Autodesk Inventor part; units mm, degrees
ref_plane "YZ Plane" through (0, 0, 0) normal (1, 0, 0) x (0, 1, 0)
ref_plane "XZ Plane" through (0, 0, 0) normal (0, 1, 0) x (-1, 0, 0)
ref_plane "XY Plane" through (0, 0, 0) normal (0, 0, 1) x (1, 0, 0)
sketch "Sketch1" plane through (0, 0, 0) normal (0, 0, 1) x (1, 0, 0)
  line L0 (0, 0) -> (58, 0)
  line L1 (58, 0) -> (58, 178)
  line L2 (58, 178) -> (0, 178)
  line L3 (0, 178) -> (0, 0)
  dimension "d0" = 58
  dimension "d1" = 178
extrude "Extrusion1" add sketch "Sketch1" along normal blind 60
shell "Shell1" thickness 3 removed faces 1 at (19.3333, 118.6667, 0)
sketch "Sketch2" plane through (0, 0, 60) normal (0, 0, 1) x (1, 0, 0)
  line L0 (3, 3) -> (55, 3)
  line L1 (3, 3) -> (8, 3)
  line L2 (8, 3) -> (8, 6.3)
  line L3 (55, 3) -> (55, 175)
  line L4 (55, 175) -> (55, 170)
  line L5 (55, 170) -> (51.7, 170)
  line L6 (48.3, 170) -> (9.7, 170)
  line L7 (8, 168.3) -> (8, 9.7)
  line L8 (9.7, 8) -> (48.3, 8)
  line L9 (50, 9.7) -> (50, 168.3)
  circle A0 centre (8, 8) radius 1.7
  line L10 (9.7, 8) -> (13, 8)
  line L11 (8, 9.7) -> (8, 13)
  line L12 (8, 13) -> (13, 13)
  line L13 (13, 13) -> (13, 8)
  line L14 (29, 8) -> (29, 9.7)
  circle A1 centre (50, 8) radius 1.7
  line L15 (48.3, 8) -> (45, 8)
  line L16 (50, 9.7) -> (50, 13)
  line L17 (50, 13) -> (45, 13)
  line L18 (45, 13) -> (45, 8)
  line L19 (50, 89) -> (45, 89)
  circle A2 centre (8, 170) radius 1.7
  line L20 (9.7, 170) -> (13, 170)
  line L21 (8, 168.3) -> (8, 165)
  line L22 (8, 165) -> (13, 165)
  line L23 (13, 165) -> (13, 170)
  circle A3 centre (50, 170) radius 1.7
  line L24 (48.3, 170) -> (45, 170)
  line L25 (50, 168.3) -> (50, 165)
  line L26 (45, 165) -> (45, 170)
  line L27 (50, 165) -> (45, 165)
  point P0 (0, 0)
  point P1 (58, 0)
  point P2 (58, 178)
  point P3 (0, 178)
  point P4 (50, 6.3)
  point P5 (8, 171.7)
  point P6 (50, 171.7)
  dimension "d29" = 5
  dimension "d31" = 5
  dimension "d32" = 5
  dimension "d33" = 3.4
  dimension "d34" = 3.3
  dimension "d35" = 3.3
extrude "Extrusion4" cut sketch "Sketch2" against normal blind 3 contours A0 | A3 | L7 L22 L23 L6 L26 L27 L9 L17 L18 L8 L13 L12 | A2 | A1
sketch "Sketch4" plane through (58, 0, 0) normal (1, 0, 0) x (0, 0, -1)
  line L0 (0, 3) -> (-57, 3)
  line L1 (0, 3) -> (-3, 3)
  line L2 (-3, 3) -> (-23, 3)
  line L3 (-23, 3) -> (-23, 103)
  line L4 (-23, 103) -> (-3, 103)
  line L5 (-3, 103) -> (-3, 3)
  line L6 (-23, 3) -> (-23, 13)
  line L7 (-23, 13) -> (-3, 13)
  point P0 (0, 0)
  dimension "d38" = 3
  dimension "d39" = 20
  dimension "d40" = 100
  dimension "d41" = 10
extrude "Extrusion5" cut sketch "Sketch4" against normal blind 4 contours L7 L3 L4 L5
sketch "Sketch5" plane through (0, 178, 0) normal (0, 1, 0) x (1, 0, 0)
  line L0 (55, 0) -> (3, 0)
  line L1 (29, 0) -> (29, -60)
  line L2 (58, -60) -> (0, -60)
  line L3 (55, 0) -> (55, -57)
  circle A0 centre (43.5, -30) radius 2.5
  circle A1 centre (14.5, -30) radius 2.5
  point P0 (0, 0)
  dimension "d44" = 5
extrude "Extrusion6" cut sketch "Sketch5" against normal blind 4
properties part number "port side"
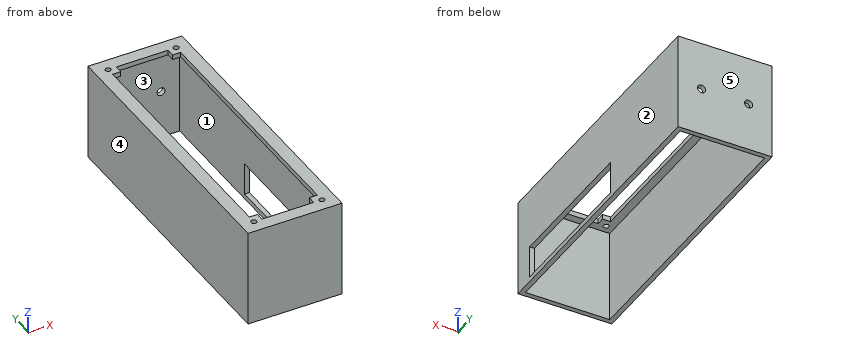
The model under review builds one solid part; all positions refer to its coordinate system, in mm. Face numbers are marked on the shaded views. A direction names the side the tool comes from. Round coordinates to 2 decimals unless told otherwise and drop trailing zeros. Loops run counter-clockwise (first coordinate to the right, second up) from the corner with the lowest first, then second, coordinate; pieces in that order, holes last. Notation, with made-up numbers: (-8.5, 74.25) - (9.5, 74.25) arc R21 cw to (9.5, 78.25) - close; hole circle Ø5 at (72, 45). An arc over 180 degrees is marked (long way). Use a Markdown table: item, result. Add a question column.
Q1. Add section D-D (x = 15). State the section outline as (y, z) points, plus the area to 3 significant figures.
Q2. For probe 1 along Y at (x, z) = (34, 45.5); probe 2 along X at (y, z) = (22, 43.5); probe 3 along X at (y, z) = (175.8, 30), list the stretches that pass through material, from the lowest coordinate up.
Q3. Machinability: for the marked faces 1 and 2, which of the approach directions +Z, -Z, +X, -X, +Y, -Y give a long, thin tool a straight path to every point of the face, cutting with its end or side? Answer none if there is none.
Q4. Add section C-C (y = 44). State the section outline as (x, z) points.
Q5. Insertion check: pin 1 Ø17 at (y, z) = (81.5, 26) entering from -X; pin 2 Ø2 at (y, z) = (57, 11.5) entering from +X; pin 3 Ø4 at (x, y) = (8, 8) entering from -Z. Each pin has a flat end and moves straight along its axis. Give the tip position at first contact, or say it passes through.
Q6. Add section A-A (y = 159). State the section outline as (x, z) points.
Q7. The part is to be moulded in two halves that separate along X. For the marked faces 3, 4 and 5, say which applies: pulls with the +X half, pulls with the -X half, needs draft (parallel to the pull), parting line crosses it, or undercut.
Q8. Add section B-B (z = 30). State the section outline as (x, y) points.
Worked answers:
| question | item | result |
|---|---|---|
| 1 | outline | (0, 0) - (3, 0) - (3, 57) - (8, 57) - (8, 60) - (0, 60) - close; (170, 57) - (175, 57) - (175, 32.45) - (178, 32.45) - (178, 60) - (170, 60) - close; (175, 0) - (178, 0) - (178, 27.55) - (175, 27.55) - close |
| 1 | area | 375 mm² |
| 2 | probe 1 | 0 to 3, 175 to 178 |
| 2 | probe 2 | 0 to 3, 55 to 58 |
| 2 | probe 3 | 0 to 12, 17 to 41, 46 to 58 |
| 3 | face 1 | -Z |
| 3 | face 2 | +Z, -Z, +X, +Y, -Y |
| 4 | outline | (0, 0) - (3, 0) - (3, 57) - (8, 57) - (8, 60) - (0, 60) - close; (50, 57) - (55, 57) - (55, 23) - (58, 23) - (58, 60) - (50, 60) - close; (55, 0) - (58, 0) - (58, 3) - (55, 3) - close |
| 5 | pin 1 | x = 0 |
| 5 | pin 2 | x = 3 |
| 5 | pin 3 | z = 57 |
| 6 | outline | (0, 0) - (3, 0) - (3, 57) - (8, 57) - (8, 60) - (0, 60) - close; (50, 57) - (55, 57) - (55, 0) - (58, 0) - (58, 60) - (50, 60) - close |
| 7 | face 3 | undercut |
| 7 | face 4 | pulls with the -X half |
| 7 | face 5 | needs draft |
| 8 | outline | (0, 0) - (58, 0) - (58, 178) - (46, 178) - (46, 175) - (55, 175) - (55, 3) - (3, 3) - (3, 175) - (12, 175) - (12, 178) - (0, 178) - close; (17, 175) - (41, 175) - (41, 178) - (17, 178) - close |
